Here's how the part is built. I have some questions about the finished solid (model axes, mm). Face numbers are marked on the shaded views. A direction names the side the tool comes from. Round coordinates to 2 decimals unless told otherwise and drop trailing zeros. Write each loop counter-clockwise with the first axis right and the second up, starting at its lowest first coordinate (ties: lowest second). Pieces come first, ordered by that corner, then holes. Notation, with made-up numbers: (32.5, -35.75) -> (62.5, -35.75) arc R21 ccw to (62.5, -7.75) -> close; hole circle Ø5 at (-3, -21.75). An arc over 180 degrees is marked (long way). Answer in a Markdown table with one row per item.
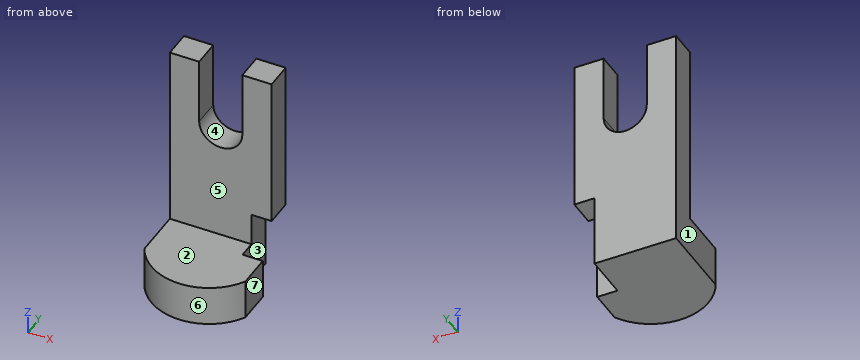
from build123d import *

# Parameters (mm, degrees)
F1_DEPTH = 12.7
F2_W     = 47.2951717675
F2_H     = 18.6941325665
F3_DEPTH = 38.354
F5_DEPTH = 25.4
F6_W     = 20.7277107984
F6_H     = 33.9597482234
F7_DEPTH = 9.398


with BuildPart() as f1:
    # F0 (on Front) → F1 (new body)
    with BuildSketch(Plane.XZ):
        with BuildLine():
            Line((-10.0103262812, 52.5179617107), (-23.6475858837, 52.5179617107))
            Line((-23.6475858837, 52.5179617107), (-23.6475858837, -52.5179617107))
            Line((-23.6475858837, -52.5179617107), (23.6475858837, -52.5179617107))
            Line((23.6475858837, -52.5179617107), (23.6475858837, 52.5179617107))
            Line((23.6475858837, 52.5179617107), (10.0103300065, 52.5179617107))
            Line((10.0103300065, 52.5179617107), (10.0103300065, 21.4714333415))
            ThreePointArc((10.0103300065, 21.4714333415), (1.8626e-06, 11.4611051977), (-10.0103262812, 21.4714333415))
            Line((-10.0103262812, 21.4714333415), (-10.0103262812, 52.5179617107))
        make_face()
    extrude(amount=F1_DEPTH)

    # F2 (on face) → F3 (join)
    with BuildSketch(Plane.XZ.offset(12.7)):
        with Locations((0, -43.1708954275)):
            Rectangle(F2_W, F2_H)
    extrude(amount=F3_DEPTH)

    # F4 (on face) → F5 (cut)
    with BuildSketch(Plane.XY.offset(-33.8238291442)):
        with BuildLine():
            ThreePointArc((23.6475858837, -36.3668836653), (-0.1790720486, -50.2147851715), (-23.6475858837, -35.7682332397))
            Line((-23.6475858837, -35.7682332397), (-23.6475858837, -51.054))
            Line((-23.6475858837, -51.054), (23.6475858837, -51.054))
            Line((23.6475858837, -51.054), (23.6475858837, -36.3668836653))
        make_face()
    extrude(amount=-F5_DEPTH, mode=Mode.SUBTRACT)

    # F6 (on face) → F7 (cut)
    with BuildSketch(Plane.YZ.offset(23.6475858837)):
        with Locations((-10.3638553992, -35.538087599)):
            Rectangle(F6_W, F6_H)
    extrude(amount=-F7_DEPTH, mode=Mode.SUBTRACT)


solid = f1.part
1) I need wall thicknesses on line 1 (X direction, y = -11, z = 40.5); line 2 (Z direction, x = -19, y = -42); line 3 (Y direction, x = 6.5, z = -16). Which ranges of each line are inside material? Lowest first, please. Write a range as [from, to].
Response:
| item | result |
|---|---|
| line 1 | x = [-23.65, -10.01], [10.01, 23.65] |
| line 2 | z = [-52.52, -33.82] |
| line 3 | y = [-12.7, 0] |
2) I want a section at D-D, the plane x = -14. List the corners of the cut face in (y, z) for me, and give its area (3 significant figures).
Response:
| item | result |
|---|---|
| outline | (-46.18, -52.52) -> (0, -52.52) -> (0, 52.52) -> (-12.7, 52.52) -> (-12.7, -33.82) -> (-46.18, -33.82) -> close |
| area | 1,960 mm^2 |
3) For pin 1 (4.5 mm diameter, centred on x = 20.5, y = -3.5, fed in from -Z); pin 2 (12 mm diameter, centred on x = -7, z = -24.5, fed in from -Y); pin 3 (5 mm diameter, centred on x = -4.5, y = -39.5, fed in from +Z), each with a flat end and sliding along its axis, tell me the tip position at first contact or that it passes through.
Response:
| item | result |
|---|---|
| pin 1 | stops at z = -18.56 |
| pin 2 | stops at y = -12.7 |
| pin 3 | stops at z = -33.82 |
4) I want a section at B-B, the plane y = -8. List the corners of the cut face in (x, z) for me.
Response:
| item | result |
|---|---|
| outline | (-23.65, -52.52) -> (14.25, -52.52) -> (14.25, -18.56) -> (23.65, -18.56) -> (23.65, 52.52) -> (10.01, 52.52) -> (10.01, 21.47) arc R10.01 cw to (-10.01, 21.47) -> (-10.01, 52.52) -> (-23.65, 52.52) -> close |
5) We'd pull the mould along X, two halves only. Please class the marked faces 4, 5, 6 and 7: +X half, -X half, draft (parallel to the pull), parting line (faces both ways), or undercut.
Response:
| item | result |
|---|---|
| face 4 | undercut |
| face 5 | draft |
| face 6 | parting line |
| face 7 | +X half |
6) I want a section at A-A, the plane z = 19. List the corners of the cut face in (x, y) for me, and give its area (3 significant figures).
Response:
| item | result |
|---|---|
| outline | (-23.65, -12.7) -> (-9.7, -12.7) -> (-9.7, 0) -> (-23.65, 0) -> close; (9.7, -12.7) -> (23.65, -12.7) -> (23.65, 0) -> (9.7, 0) -> close |
| area | 354 mm^2 |
7) Which directions (+Z, -Z, +X, -X, +Y, -Y) give clear straight access to the entire face, cutting with the end or side of a thin tool? Please do the marked faces 1, 2 and 3.
Response:
| item | result |
|---|---|
| face 1 | +Z, -Z, -X, +Y, -Y |
| face 2 | +Z, +X, -X, -Y |
| face 3 | -Z, +X, +Y |
8) I want a section at C-C, the plane z = -40.5. List the corners of the cut face in (x, y) for me.
Response:
| item | result |
|---|---|
| outline | (-23.65, -35.77) arc R26.84 ccw to (23.65, -36.37) -> (23.65, -20.73) -> (14.25, -20.73) -> (14.25, 0) -> (-23.65, 0) -> close |
